Geometry check sheet. Reference: the model listing, model coordinates, mm. Face numbers are marked on the shaded views. A direction names the side the tool comes from. Give positions to 0.01 mm unless a question says otherwise; leave off trailing zeros. Order: outer loops, then holes, each group sorted by start corner. A loop starts at its lowest first (then second) coordinate and runs counter-clockwise, first axis right, second up. Notation, with made-up numbers: M 41.5,-23 L 74.5,-23 A7 cw 74.5,-14 Z; hole C 38.25,-34.5 d10. An arc over 180 degrees is marked long. Use CSV: the item, a comma, the result in double quotes. Start each with the question number.
from build123d import *

# Parameters (mm, degrees)
ESQUISSE1_R             = 31.5
ESQUISSE1_R_2           = 22.5
BOSS_EXTRU_1_DEPTH      = 20
ENL_V_MAT_EXTRU_1_DEPTH = 21
BOSS_EXTRU_2_DEPTH      = 20
ESQUISSE4_R             = 22.5
BOSS_EXTRU_3_DEPTH      = 4.5
ENL_V_MAT_EXTRU_2_REACH = 6.5
ESQUISSE5_R             = 2
ESQUISSE6_W             = 9
ESQUISSE6_H             = 5


with BuildPart() as part:
    # Esquisse1 → Boss.-Extru.1 (new body)
    with BuildSketch(Plane(origin=(0, 0, 0), x_dir=(1, 0, 0), z_dir=(0, 1, 0))):
        Circle(ESQUISSE1_R)
        Circle(ESQUISSE1_R_2, mode=Mode.SUBTRACT)
    extrude(amount=BOSS_EXTRU_1_DEPTH)

    # Esquisse2 → Enlèv. mat.-Extru.1 (cut, through all)
    with BuildSketch(Plane(origin=(0, 20, 0), x_dir=(1, 0, 0), z_dir=(0, 1, 0))):
        with BuildLine():
            ThreePointArc((-15.75, 27.279800219), (-27.279800219, 15.75), (-31.5, 0))
            ThreePointArc((-31.5, 0), (-29.25, -2.25), (-27, 0))
            ThreePointArc((-27, 0), (-23.382685902, 13.5), (-13.5, 23.382685902))
            ThreePointArc((-13.5, 23.382685902), (-12.676442841, 26.456243061), (-15.75, 27.279800219))
        make_face()
        with BuildLine():
            ThreePointArc((31.5, 0), (27.279800219, 15.75), (15.75, 27.279800219))
            ThreePointArc((15.75, 27.279800219), (12.676442841, 26.456243061), (13.5, 23.382685902))
            ThreePointArc((13.5, 23.382685902), (23.382685902, 13.5), (27, 0))
            ThreePointArc((27, 0), (29.25, -2.25), (31.5, 0))
        make_face()
        with BuildLine():
            ThreePointArc((-15.75, -27.279800219), (0, -31.5), (15.75, -27.279800219))
            ThreePointArc((15.75, -27.279800219), (16.573557159, -24.206243061), (13.5, -23.382685902))
            ThreePointArc((13.5, -23.382685902), (0, -27), (-13.5, -23.382685902))
            ThreePointArc((-13.5, -23.382685902), (-16.573557159, -24.206243061), (-15.75, -27.279800219))
        make_face()
    extrude(amount=-ENL_V_MAT_EXTRU_1_DEPTH, mode=Mode.SUBTRACT)

    # Esquisse3 → Boss.-Extru.2 (add)
    with BuildSketch(Plane(origin=(0, 20, 0), x_dir=(1, 0, 0), z_dir=(0, 1, 0))):
        with BuildLine():
            ThreePointArc((25.455844123, 25.455844123), (0, 36), (-25.455844123, 25.455844123))
            ThreePointArc((-25.455844123, 25.455844123), (-25.455844123, 22.273863607), (-22.273863607, 22.273863607))
            ThreePointArc((-22.273863607, 22.273863607), (0, 31.5), (22.273863607, 22.273863607))
            ThreePointArc((22.273863607, 22.273863607), (25.455844123, 22.273863607), (25.455844123, 25.455844123))
        make_face()
        with BuildLine():
            ThreePointArc((9.317485624, -34.773329746), (31.176914536, -18), (34.773329746, 9.317485624))
            ThreePointArc((34.773329746, 9.317485624), (32.017653786, 10.908475881), (30.426663528, 8.152799921))
            ThreePointArc((30.426663528, 8.152799921), (27.279800219, -15.75), (8.152799921, -30.426663528))
            ThreePointArc((8.152799921, -30.426663528), (6.561809663, -33.182339489), (9.317485624, -34.773329746))
        make_face()
        with BuildLine():
            ThreePointArc((-34.773329746, 9.317485624), (-31.176914536, -18), (-9.317485624, -34.773329746))
            ThreePointArc((-9.317485624, -34.773329746), (-6.561809663, -33.182339489), (-8.152799921, -30.426663528))
            ThreePointArc((-8.152799921, -30.426663528), (-27.279800219, -15.75), (-30.426663528, 8.152799921))
            ThreePointArc((-30.426663528, 8.152799921), (-32.017653786, 10.908475881), (-34.773329746, 9.317485624))
        make_face()
    extrude(amount=-BOSS_EXTRU_2_DEPTH)

    # Esquisse4 → Boss.-Extru.3 (add)
    with BuildSketch(Plane.XZ):
        Circle(ESQUISSE4_R)
    extrude(amount=-BOSS_EXTRU_3_DEPTH)

    # Esquisse5 → Enlèv. mat.-Extru.2 (cut, up to next)
    with BuildSketch(Plane(origin=(0, 4.5, 0), x_dir=(1, 0, 0), z_dir=(0, 1, 0)), mode=Mode.PRIVATE) as enl_v_mat_extru_2_sk1:
        with Locations((0, 16)):
            Circle(ESQUISSE5_R)
    enl_v_mat_extru_2_tool1 = extrude(enl_v_mat_extru_2_sk1.sketch, amount=-ENL_V_MAT_EXTRU_2_REACH, mode=Mode.PRIVATE) & part.part
    add(enl_v_mat_extru_2_tool1.solids().sort_by_distance((0, 4.5, -16))[0], mode=Mode.SUBTRACT)
    # Esquisse5 → Enlèv. mat.-Extru.2 (cut, up to next)
    with BuildSketch(Plane(origin=(0, 4.5, 0), x_dir=(1, 0, 0), z_dir=(0, 1, 0)), mode=Mode.PRIVATE) as enl_v_mat_extru_2_sk2:
        with Locations((13.856406461, -8)):
            Circle(ESQUISSE5_R)
    enl_v_mat_extru_2_tool2 = extrude(enl_v_mat_extru_2_sk2.sketch, amount=-ENL_V_MAT_EXTRU_2_REACH, mode=Mode.PRIVATE) & part.part
    add(enl_v_mat_extru_2_tool2.solids().sort_by_distance((13.856406, 4.5, 8))[0], mode=Mode.SUBTRACT)
    # Esquisse5 → Enlèv. mat.-Extru.2 (cut, up to next)
    with BuildSketch(Plane(origin=(0, 4.5, 0), x_dir=(1, 0, 0), z_dir=(0, 1, 0)), mode=Mode.PRIVATE) as enl_v_mat_extru_2_sk3:
        with Locations((-13.856406461, -8)):
            Circle(ESQUISSE5_R)
    enl_v_mat_extru_2_tool3 = extrude(enl_v_mat_extru_2_sk3.sketch, amount=-ENL_V_MAT_EXTRU_2_REACH, mode=Mode.PRIVATE) & part.part
    add(enl_v_mat_extru_2_tool3.solids().sort_by_distance((-13.856406, 4.5, 8))[0], mode=Mode.SUBTRACT)

    # Esquisse6 → Enlèvement de matière-Révolution1 (revolve, cut)
    with BuildSketch(Plane(origin=(0, 0, 0), x_dir=(0, 0, -1), z_dir=(1, 0, 0))):
        with Locations((31.5, 10)):
            Rectangle(ESQUISSE6_W, ESQUISSE6_H)
    revolve(axis=Axis((0, 10, 0), (0, -1, 0)), mode=Mode.SUBTRACT)


solid = part.part
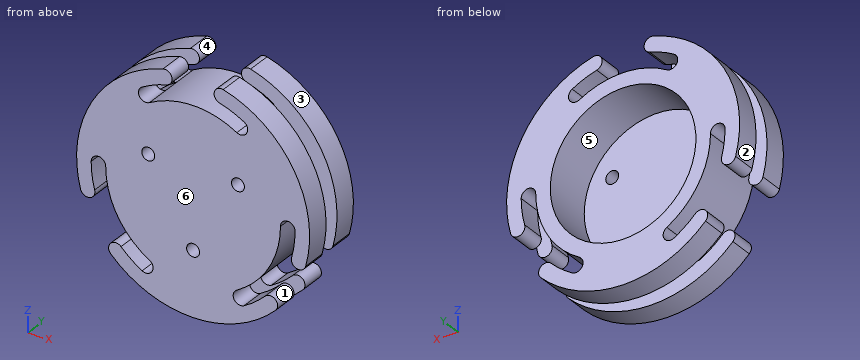
(1) Draft check along X on the marked faces 1, 2, 3 and 4. Enter one of: +X half, -X half, draft (parallel to the pull), parting line (faces both ways), or undercut.
(2) Access from +Z, -Z, +X, -X, +Y, -Y to the whole of each face (thin tool, end or side, straight path). Record for the marked faces 5 and 6.
(3) Sectioned sample at A-A on x = 0. Record the cut outline in (y, z), then the cut area to 4 significant figures.
(4) Thickness scan on line 1 (Z direction, x = 0, y = 2.4); line 2 (Y direction, x = -6, z = -30); line 3 (Z direction, x = 13, y = 7) (3 decimals). Record the ranges inside material, lowest first.
(5) Sectioned sample at C-C on y = 17.5. Record the cut outline in (x, z) (3 decimals).
(6) Go/stop test with flat-tipped pins: P1, Ø6, axis at x = -26.5, y = 16.5, coming from the +Z side; P2, Ø8, axis at x = 6, z = 12, coming from the +Y side; P3, Ø2, axis at x = 20, y = 15, coming from the -Z side; P4, Ø4, axis at x = -24, z = 9, coming from the -Y side. Record where each tip stops, or that it passes through.
(7) Sectioned sample at B-B on z = 8. Record the cut outline in (x, y).
(8) Sectioned sample at D-D on z = -17. Record the cut outline in (x, y), then the cut area to 3 significant figures.
Responses:
1,face 1,"undercut"
1,face 2,"-X half"
1,face 3,"+X half"
1,face 4,"undercut"
2,face 5,"+Y"
2,face 6,"+Z, -Z, +X, -X, -Y"
3,outline,"M 0,-36 L 7.5,-36 L 7.5,-27 L 12.5,-27 L 12.5,-36 L 20,-36 L 20,-22.5 L 4.5,-22.5 L 4.5,-18 L 0,-18 Z; M 0,-14 L 4.5,-14 L 4.5,22.5 L 20,22.5 L 20,27 L 0,27 Z"
3,area,"499.5 mm2"
4,line 1,"-36 to -18, -14 to 27"
4,line 2,"0 to 7.5, 12.5 to 20"
4,line 3,"-33.571 to -26.887, -23.775 to -18.364, 18.364 to 23.664, 28.692 to 33.571"
5,outline,"M -34.773,-9.317 A2.25 ccw -30.427,-8.153 A31.5 cw -31.5,0 A2.25 cw -27,0 A27 ccw -13.5,-23.383 A2.25 cw -15.75,-27.28 A31.5 cw -22.274,-22.274 A2.25 ccw -25.456,-25.456 A36 ccw 25.456,-25.456 A2.25 ccw 22.274,-22.274 A31.5 cw 15.75,-27.28 A2.25 cw 13.5,-23.383 A27 ccw 27,0 A2.25 cw 31.5,0 A31.5 cw 30.427,-8.153 A2.25 ccw 34.773,-9.317 A36 ccw 9.317,34.773 A2.25 ccw 8.153,30.427 A31.5 cw 15.75,27.28 A2.25 cw 13.5,23.383 A27 ccw -13.5,23.383 A2.25 cw -15.75,27.28 A31.5 cw -8.153,30.427 A2.25 ccw -9.317,34.773 A36 ccw Z; hole C 0,0 d45"
6,P1,"z = 27.27"
6,P2,"y = 4.5"
6,P3,"z = -30.58"
6,P4,"y = 0"
7,outline,"M -35.1,0 L -15.86,0 L -15.86,4.5 L -21.03,4.5 L -21.03,20 L -35.1,20 L -35.1,12.5 L -25.79,12.5 L -25.79,7.5 L -35.1,7.5 Z; M -11.86,0 L 11.86,0 L 11.86,4.5 L -11.86,4.5 Z; M 15.86,0 L 35.1,0 L 35.1,7.5 L 25.79,7.5 L 25.79,12.5 L 35.1,12.5 L 35.1,20 L 21.03,20 L 21.03,4.5 L 15.86,4.5 Z"
8,outline,"M -20.98,0 L -1.73,0 L -1.73,4.5 L -14.74,4.5 L -14.74,20 L -20.98,20 Z; M 1.73,0 L 20.98,0 L 20.98,20 L 14.74,20 L 14.74,4.5 L 1.73,4.5 Z"
8,area,"367 mm2"
